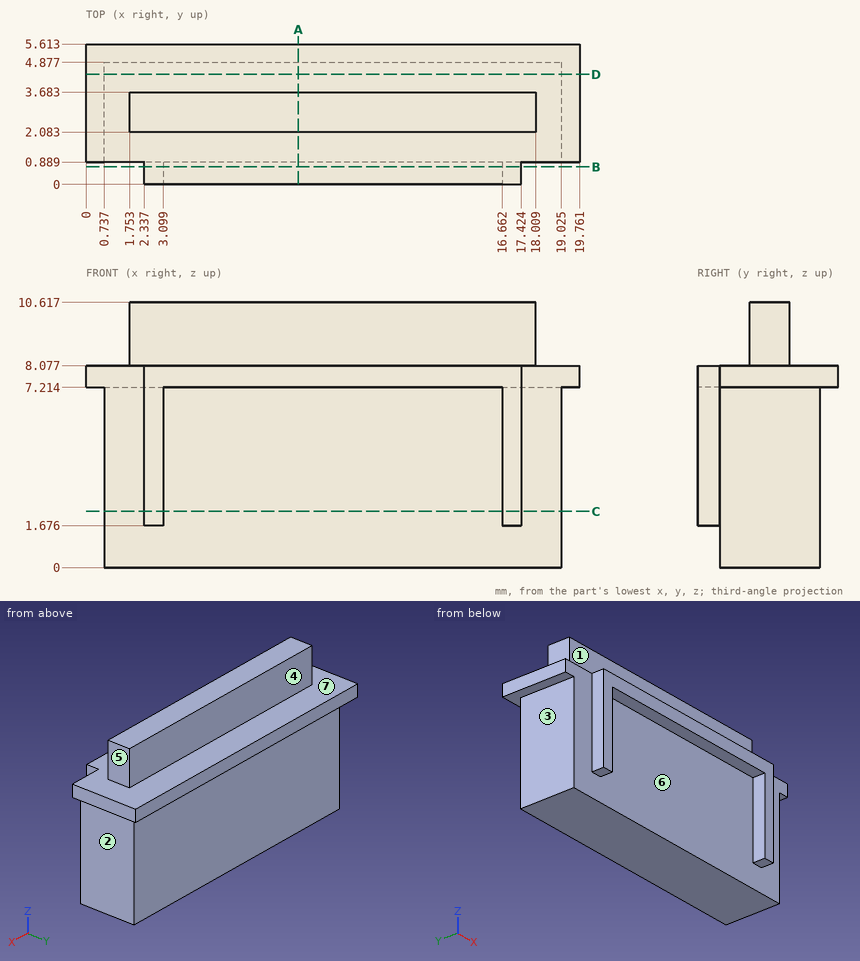
Check sheet for the drawn part. Datum: minimum x, y, z corner. Units: mm. A direction names the side the tool comes from. Round coordinates to 2 decimals unless told otherwise and drop trailing zeros. Loops run counter-clockwise (first coordinate to the right, second up) from the corner with the lowest first, then second, coordinate; pieces in that order, holes last.
Item 1: Cross-section at B-B on y = 0.7. Record the boundary of the cut face in (x, z) (1 decimal).
Item 2: Cross-section at D-D on y = 4.4. Record the boundary of the cut face in (x, z) (1 decimal), then the cut area to 3 significant figures.
Item 3: Mould release check, pull along X, two halves, no side actions. Record for the marked faces 5, 6 and 7: pulls with the +X half, pulls with the -X half, needs draft (parallel to the pull), parting line crosses it, or undercut.
Item 4: Cross-section at A-A on x = 8.5. Record the boundary of the cut face in (y, z).
Item 5: Thickness scan on line 1 (Z direction, x = 6.5, y = 5.2); line 2 (Y direction, x = 15.5, z = 9.25); line 3 (X direction, y = 1.85, z = 4.75) (1 decimal). Record the ranges inside material, lowest first.
Item 6: Access from +Z, -Z, +X, -X, +Y, -Y to the whole of each face (thin tool, end or side, straight path). Record for the marked faces 1, 2, 3 and 4.
Item 7: Gauge pin test, flat ends, axial feed: pin 1 (1.2 mm diameter, centred on y = 3, z = 3.5, fed in from -X); pin 2 (5 mm diameter, centred on x = 9.5, z = 5.5, fed in from -Y); pin 3 (1 mm diameter, centred on y = 3, z = 6, fed in from +X) (1 decimal); pin 4 (0.8 mm diameter, centred on x = 7, z = 9, fed in from -Y). Record the tip position at first contact, or that the pin passes through.
Item 8: Cross-section at C-C on z = 2.25. Record the boundary of the cut face in (x, y) (1 decimal).
Answer sheet:
1. outline: (2.3, 1.7) - (3.1, 1.7) - (3.1, 7.2) - (16.7, 7.2) - (16.7, 1.7) - (17.4, 1.7) - (17.4, 8.1) - (2.3, 8.1) - close
2. outline: (0, 7.2) - (0.7, 7.2) - (0.7, 0) - (19, 0) - (19, 7.2) - (19.8, 7.2) - (19.8, 8.1) - (0, 8.1) - close
2. area: 149 mm2
3. face 5: pulls with the +X half
3. face 6: undercut
3. face 7: needs draft
4. outline: (0, 7.21) - (0.89, 7.21) - (0.89, 0) - (4.88, 0) - (4.88, 7.21) - (5.61, 7.21) - (5.61, 8.08) - (3.68, 8.08) - (3.68, 10.62) - (2.08, 10.62) - (2.08, 8.08) - (0, 8.08) - close
5. line 1: z = 7.21 to 8.08
5. line 2: y = 2.08 to 3.68
5. line 3: x = 0.7 to 19
6. face 1: +Z, +X, -X, -Y
6. face 2: -Z, +X, +Y, -Y
6. face 3: -Z, -X, +Y, -Y
6. face 4: +Z, +X, -X, +Y
7. pin 1: stops at x = 0.74
7. pin 2: stops at y = 0
7. pin 3: stops at x = 19
7. pin 4: stops at y = 2.08
8. outline: (0.7, 0.9) - (2.3, 0.9) - (2.3, 0) - (3.1, 0) - (3.1, 0.9) - (16.7, 0.9) - (16.7, 0) - (17.4, 0) - (17.4, 0.9) - (19, 0.9) - (19, 4.9) - (0.7, 4.9) - close
